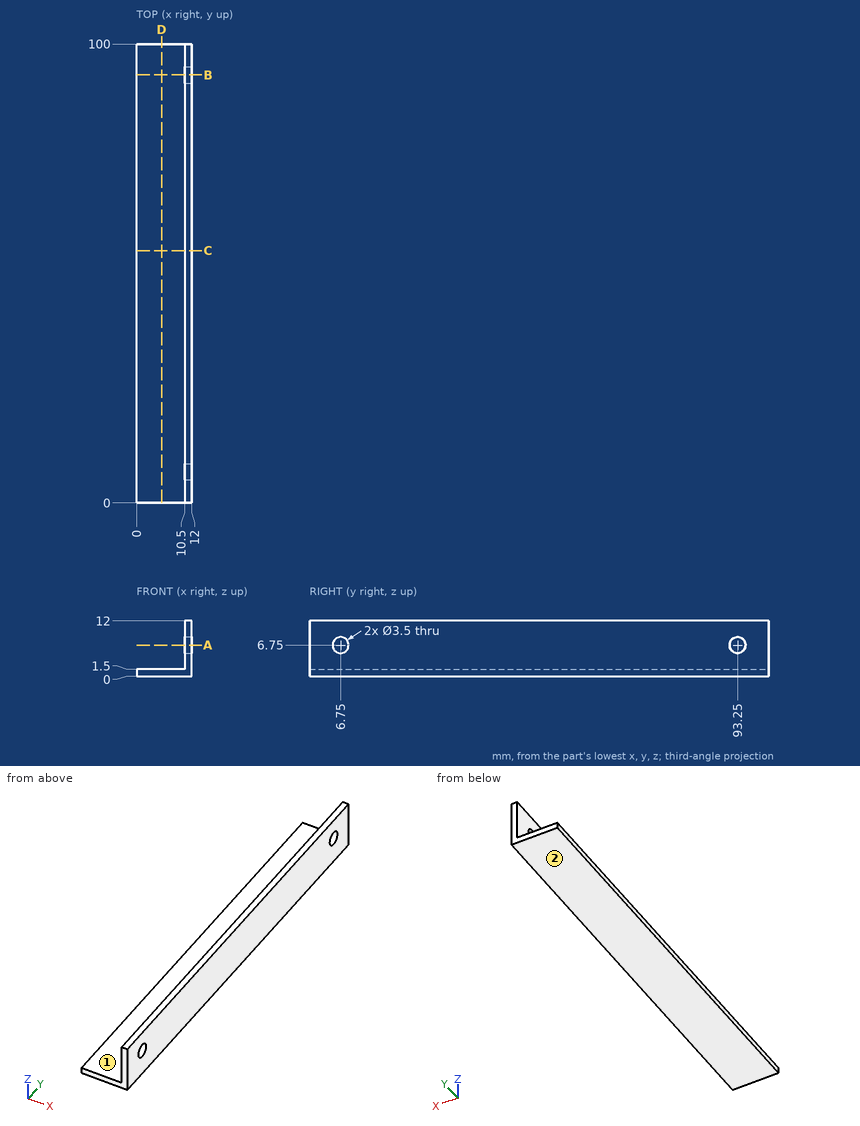
Here's the drawing with two shaded views (mm, measured from the low corner). I have some questions. A direction names the side the tool comes from. Round coordinates to 2 decimals unless told otherwise and drop trailing zeros. Write each loop counter-clockwise with the first axis right and the second up, starting at its lowest first coordinate (ties: lowest second). Pieces come first, ordered by that corner, then holes. Notation, with made-up numbers: M 20.5,-25.75 L 64.5,-25.75 A9 ccw 64.5,-14.75 Z; hole C -8.5,86.5 d1. An arc over 180 degrees is marked long. Use CSV: the item, a comma, the result in double quotes.
(1) On a 3-axis mill with a long thin cutter (end or side, diameter ignored), from which of +Z, -Z, +X, -X, +Y, -Y can I reach the whole of each face in a straight line? I mean the marked faces 1 and 2. Say none if no direction works.
Check values:
face 1,"+Z, -X, +Y, -Y"
face 2,"-Z, +X, -X, +Y, -Y"
(2) Imagine slicing it at C-C (y = 55). Write out the boundary of the cut face in (x, z), plus the area to 4 significant figures.
Check values:
outline,"M 0,0 L 12,0 L 12,12 L 10.5,12 L 10.5,1.5 L 0,1.5 Z"
area,"33.75 mm^2"
(3) Imagine slicing it at B-B (y = 93.25). Write out the boundary of the cut face in (x, z).
Check values:
outline,"M 0,0 L 12,0 L 12,5 L 10.5,5 L 10.5,1.5 L 0,1.5 Z; M 10.5,8.5 L 12,8.5 L 12,12 L 10.5,12 Z"
(4) I need wall thicknesses on line 1 along Y through (x, z) = (11, 6.75); line 2 along Z through (x, y) = (10.85, 93.25); line 3 along X through (y, z) = (69.5, 10). Which ranges of each line are inside material? Lowest first, please.
Check values:
line 1,"0 to 5, 8.5 to 91.5, 95 to 100"
line 2,"0 to 5, 8.5 to 12"
line 3,"10.5 to 12"
(5) Imagine slicing it at D-D (x = 5.5). Write out the boundary of the cut face in (y, z), plus the area to 3 significant figures.
Check values:
outline,"M 0,0 L 100,0 L 100,1.5 L 0,1.5 Z"
area,"150 mm^2"
(6) I'm going to push a flat-ended pin straight in: pin 1 (1 mm diameter, centred on x = 6.5, y = 45, fed in from +Z). Where does the tip first touch, or does it pass through?
Check values:
pin 1,"z = 1.5"
(7) Imagine slicing it at A-A (z = 6.75). Write out the boundary of the cut face in (x, y), plus the area to 4 significant figures.
Check values:
outline,"M 10.5,0 L 12,0 L 12,5 L 10.5,5 Z; M 10.5,8.5 L 12,8.5 L 12,91.5 L 10.5,91.5 Z; M 10.5,95 L 12,95 L 12,100 L 10.5,100 Z"
area,"139.5 mm^2"
